The listing builds one solid part. Answer for the finished solid, in the listing's coordinates (mm). Coordinates: 2 decimals unless noted, no trailing zeros. Loops run counter-clockwise (first coordinate to the right, second up) from the corner with the lowest first, then second, coordinate; pieces in that order, holes last. Notation, with made-up numbers: (-3.75, 29) - (14.25, 29) arc R10 cw to (14.25, 33) - close; hole circle Ø4 at (-33, 2). An arc over 180 degrees is marked (long way). One line per question, with ' | ' between items.
from build123d import *

# Parameters (mm, degrees)
F0_W     = 19.05
F0_H     = 19.05
F0_R     = 5.55625
F1_DEPTH = 44.45
F3_D     = 8.4328
F5_D     = 8.4328


# Not quite as in the source:
# - a feature names something its author has since deleted; it is built from what else it names


with BuildPart() as f1:
    # F0 (on Front) → F1 (new body)
    with BuildSketch(Plane.XZ):
        with Locations((9.525, 9.525)):
            Rectangle(F0_W, F0_H)
        with Locations((9.525, 9.525)):
            Circle(F0_R, mode=Mode.SUBTRACT)
    extrude(amount=F1_DEPTH)

    # F3 (through all)
    with Locations(Plane.XY.offset(19.05)):
        with Locations((9.525, -29.21)):
            Hole(F3_D / 2)

    # F5 (through all)
    with Locations(Plane.YZ.offset(19.05)):
        with Locations((-15.24, 9.525)):
            Hole(F5_D / 2)


solid = f1.part
Item 1: Find section D-D, the plane z = 6.5. Write down the section's boundary in (x, y), plus the area to 3 significant figures.
Taken from the geometry:
outline: (0, -44.45) - (4.86, -44.45) - (4.86, -18.18) - (0, -18.18) - close; (0, -12.3) - (4.86, -12.3) - (4.86, 0) - (0, 0) - close; (14.19, -44.45) - (19.05, -44.45) - (19.05, -18.18) - (14.19, -18.18) - close; (14.19, -12.3) - (19.05, -12.3) - (19.05, 0) - (14.19, 0) - close | area: 375 mm2
Item 2: Find the intervals of material crossed by line 1 (X direction, y = -29.21, z = 15.45); line 2 (Y direction, x = 16.75, z = 6.5), in increasing order. Write a range as [from, to].
Taken from the geometry:
line 1: x = [0, 5.31], [13.74, 19.05] | line 2: y = [-44.45, -18.18], [-12.3, 0]
Item 3: This flat-tipped pin is pushed along its axis until it touches: pin 1 Ø5 at (x, y) = (9.525, -29.21) entering from -Z. Where does it stop, or does it pass through?
Taken from the geometry:
pin 1: passes through
Item 4: Find section B-B, the plane x = 14.5. Write down the section's boundary in (y, z) (3 decimals).
Taken from the geometry:
outline: (-44.45, 0) - (0, 0) - (0, 7.051) - (-11.826, 7.051) arc R4.216 cw to (-18.654, 7.051) - (-44.45, 7.051) - close; (-44.45, 11.999) - (-18.654, 11.999) arc R4.216 cw to (-11.826, 11.999) - (0, 11.999) - (0, 19.05) - (-44.45, 19.05) - close
Item 5: The mould has two halves that part along Z. Classify faces 1 (the face through (9, -22, 19.05)), 2 (the face through (14, -44.45, 14)), 3 (the face through (3.974, -21.914, 9.769)), 4 (the face through (2.256, -11.028, 9.71)): pulls with the +Z half, pulls with the -Z half, needs draft (parallel to the pull), parting line crosses it, or undercut.
Taken from the geometry:
face 1: pulls with the +Z half | face 2: needs draft | face 3: undercut | face 4: undercut
Item 6: Find section C-C, the plane z = 1.5. Write down the section's boundary in (x, y) (3 decimals), plus the area to 3 significant figures.
Taken from the geometry:
outline: (0, -44.45) - (19.05, -44.45) - (19.05, 0) - (0, 0) - close; hole circle Ø8.433 at (9.525, -29.21) | area: 791 mm2
